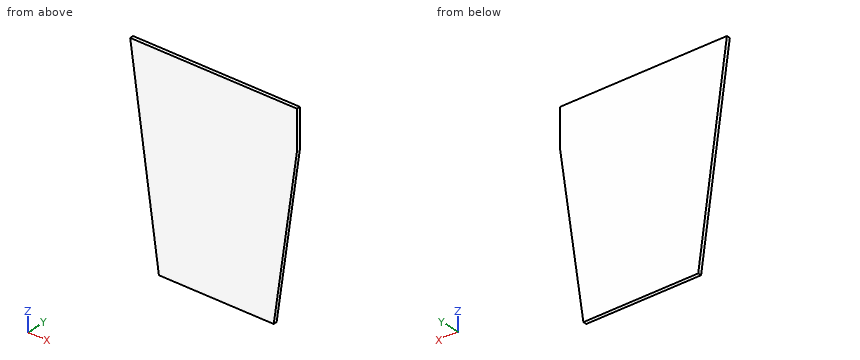
```python
from build123d import *

# Parameters (mm, degrees)
EXTRUDE_1_DEPTH     = 1.8
SKETCH_2_W          = 2.788461538
SKETCH_2_H          = 20
CUT_EXTRUDE_1_DEPTH = 136.603244799


with BuildPart() as part:
    # 草图1 → 凸台-拉伸1 (new body)
    with BuildSketch(Plane(origin=(0, 0, 0), x_dir=(1, 0, 0), z_dir=(0, 1, 0))):
        Polygon((0, 0), (14.5, 104), (72.5, 104), (87, 0), align=None)
    extrude(amount=EXTRUDE_1_DEPTH)

    # 草图2 → 切除-拉伸1 (cut, through all)
    with BuildSketch(Plane(origin=(0, 1.8, 0), x_dir=(1, 0, 0), z_dir=(0, 1, 0))):
        with Locations((85.605769231, 10)):
            Rectangle(SKETCH_2_W, SKETCH_2_H)
    extrude(amount=-CUT_EXTRUDE_1_DEPTH, mode=Mode.SUBTRACT)


solid = part.part
```
Geometry: final body of the model. Coordinates: model frame, mm. Round coordinates to 2 decimals unless told otherwise and drop trailing zeros. Write each loop counter-clockwise with the first axis right and the second up, starting at its lowest first coordinate (ties: lowest second). Pieces come first, ordered by that corner, then holes. Notation, with made-up numbers: M -19.75,46.25 L -7.75,46.25 A21 cw -7.75,65.25 Z; hole C 12,84.25 d7. An arc over 180 degrees is marked long. Answer in a Markdown table with one row per item. Add a question column.
(1) Ray query, L1, parallel to X at y = 1.5, z = -85; L2, parallel to X at y = 1.55, z = -88. Return the intervals inside material, ascending.
(2) Cut plane A-A, the plane y = 0.4. Return the cut outline in (x, z), then the cut area to 3 significant figures.
(3) Cut plane B-B, the plane z = -87. Return the cut outline in (x, y).
(4) Cut plane C-C, the plane x = 74. Return the cut outline in (y, z), then the cut area to 3 significant figures.
Established:
| question | item | result |
|---|---|---|
| 1 | L1 | 11.85 to 75.15 |
| 1 | L2 | 12.27 to 74.73 |
| 2 | outline | M 0,0 L 14.5,-104 L 72.5,-104 L 84.21,-20 L 84.21,0 Z |
| 2 | area | 7,510 mm² |
| 3 | outline | M 12.13,0 L 74.87,0 L 74.87,1.8 L 12.13,1.8 Z |
| 4 | outline | M 0,-93.24 L 1.8,-93.24 L 1.8,0 L 0,0 Z |
| 4 | area | 168 mm² |
